Build history of the part. All positions in model axes, mm. Face numbers are marked on the shaded views. A direction names the side the tool comes from. Round coordinates to 2 decimals unless told otherwise and drop trailing zeros. Loops run counter-clockwise (first coordinate to the right, second up) from the corner with the lowest first, then second, coordinate; pieces in that order, holes last. Notation, with made-up numbers: (84, 22.5) - (136, 22.5) arc R27 cw to (136, 56.5) - close; hole circle Ø3 at (37.5, -31). An arc over 180 degrees is marked (long way). Use one line per item in the form item = value. Start each with the question number.
Q1. Drill centre lines: line 1 (Z direction, x = 12.75, y = 17.5); line 2 (Z direction, x = 2.25, y = 11.5); line 3 (X direction, y = 2, z = 2.5). Where is each one in solid material? Low to high.
Q2. Pin check, flat tips, straight feed: pin 1 (2 mm diameter, centred on x = 24, z = 6, fed in from +Y); pin 2 (7.5 mm diameter, centred on x = 8, y = 18.5, fed in from +Z); pin 3 (3.5 mm diameter, centred on y = 6.5, z = 6, fed in from +X). Stop position of each tip, or through.
Q3. Mould opens along X. For the marked faces 3, 4, 5 and 6 say: released by +X, released by -X, zero draft, split by the parting line, or undercut.
Q4. Saw through at A-A (z = 5.5). Give the cut face in (x, y).
Q5. Saw through at D-D (y = 13). Give the cut face in (x, z), then the cut area to 3 significant figures.
Q6. Saw through at C-C (x = 24.5). Give the cut face in (y, z), then the cut area to 3 significant figures.
Q7. 3-axis set-ups, long thin cutter, end or side, ignore diameter. For the marked faces 1 and 2: which of +Z, -Z, +X, -X, +Y, -Y reach the whole face in a straight line?
```python
from build123d import *

# Parameters (mm, degrees)
SKETCH1_W           = 30
SKETCH1_H           = 25
BOSS_EXTRUDE1_DEPTH = 4
SKETCH3_W           = 9.7
SKETCH3_H           = 20
CUT_EXTRUDE1_DEPTH  = 1.2
FILLET1_R           = 3
SKETCH4_W           = 2
SKETCH4_H           = 7.755081554
BOSS_EXTRUDE2_DEPTH = 4
FILLET2_R           = 1


with BuildPart() as part:
    # Sketch1 → Boss-Extrude1 (new body)
    with BuildSketch(Plane.XY):
        with Locations((15, 12.5)):
            Rectangle(SKETCH1_W, SKETCH1_H)
    extrude(amount=BOSS_EXTRUDE1_DEPTH)

    # Sketch3 → Cut-Extrude1 (cut)
    with BuildSketch(Plane.XY.offset(4)):
        with Locations((15, 10)):
            Rectangle(SKETCH3_W, SKETCH3_H)
    extrude(amount=-CUT_EXTRUDE1_DEPTH, mode=Mode.SUBTRACT)

    # Fillet1
    fillet1_edges = [part.edges().sort_by_distance(p)[0] for p in [
        (0, 25, 2),
        (30, 25, 2),
        (30, 0, 2),
        (0, 0, 2),
    ]]
    fillet(fillet1_edges, radius=FILLET1_R)

    # Sketch4 → Boss-Extrude2 (add)
    with BuildSketch(Plane.XY.offset(4)):
        with Locations((24.15, 3.877540777)):
            Rectangle(SKETCH4_W, SKETCH4_H)
        with Locations((5.85, 3.877540777)):
            Rectangle(SKETCH4_W, SKETCH4_H)
    extrude(amount=BOSS_EXTRUDE2_DEPTH)

    # Fillet2
    fillet2_edges = [part.edges().sort_by_distance(p)[0] for p in [
        (25.15, 3.877540777, 4),
        (24.15, 7.755081554, 4),
        (23.15, 3.877540777, 8),
        (24.15, 0, 8),
        (25.15, 3.877540777, 8),
        (24.15, 7.755081554, 8),
        (5.85, 7.755081554, 4),
        (4.85, 3.877540777, 4),
        (6.85, 3.877540777, 8),
        (5.85, 7.755081554, 8),
        (4.85, 3.877540777, 8),
        (5.85, 0, 8),
    ]]
    fillet(fillet2_edges, radius=FILLET2_R - 0.0001)  # a hair under: the kernel refuses the full size


solid = part.part
```
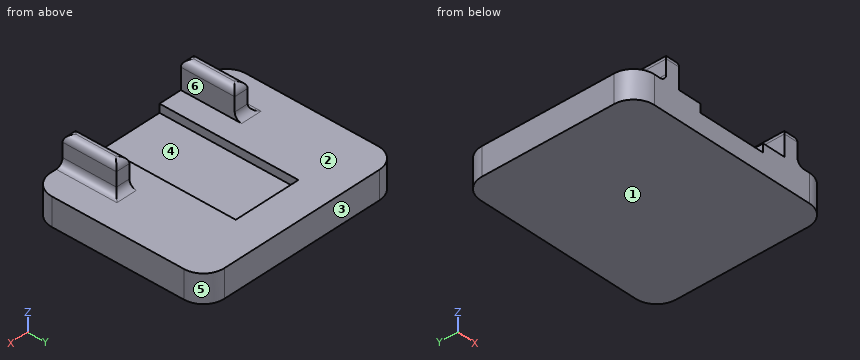
Report:
q1.line_1 = 0 to 2.8
q1.line_2 = 0 to 4
q1.line_3 = 0.17 to 29.83
q2.pin_1 = 7.76
q2.pin_2 = 4
q2.pin_3 = 25.49
q3.face_3 = zero draft
q3.face_4 = undercut
q3.face_5 = released by +X
q3.face_6 = undercut
q4.outline = (4.85, 0) - (6.85, 0) - (6.85, 7.76) - (4.85, 7.76) - close; (23.15, 0) - (25.15, 0) - (25.15, 7.76) - (23.15, 7.76) - close
q5.outline = (0, 0) - (30, 0) - (30, 4) - (19.85, 4) - (19.85, 2.8) - (10.15, 2.8) - (10.15, 4) - (0, 4) - close
q5.area = 108 mm²
q6.outline = (0, 0) - (25, 0) - (25, 4) - (8.75, 4) arc R1 cw to (7.76, 5) - (7.76, 7) arc R1 ccw to (7.11, 7.94) - (0.65, 7.94) arc R1 ccw to (0, 7) - close
q6.area = 130 mm²
q7.face_1 = -Z, +X, -X, +Y, -Y
q7.face_2 = +Z, +Y
